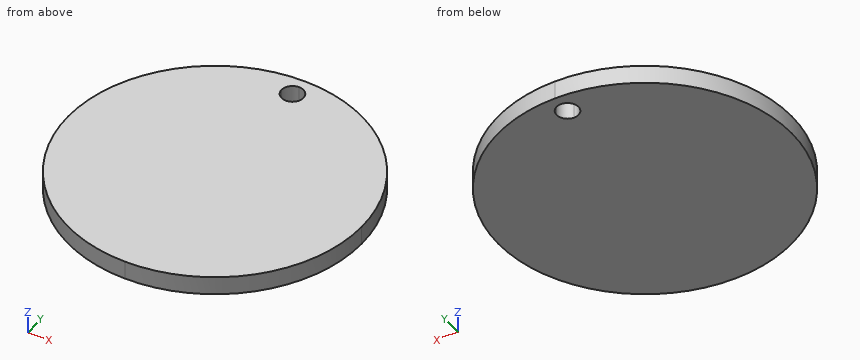
```python
from build123d import *

# Parameters (mm, degrees)
F1_DEPTH = 6.35


with BuildPart() as f1:
    # F0 (on Top) → F1 (new body)
    with BuildSketch(Plane.XY):
        with BuildLine():
            Line((0, 47.5154318641), (0, 50.8))
            ThreePointArc((0, 50.8), (-50.8, 0), (0, -50.8))
            Line((0, -50.8), (0, 39.9495042134))
            ThreePointArc((0, 39.9495042134), (-2.6749593739, 41.0575086649), (-3.7829638253, 43.7324680388))
            ThreePointArc((-3.7829638253, 43.7324680388), (-2.6749593739, 46.4074274127), (0, 47.5154318641))
        make_face()
        with BuildLine():
            ThreePointArc((0, -50.8), (35.9210244843, -35.9210244843), (50.8, 0))
            ThreePointArc((50.8, 0), (35.9210244843, 35.9210244843), (0, 50.8))
            Line((0, 50.8), (0, 47.5154318641))
            ThreePointArc((0, 47.5154318641), (2.6749593739, 46.4074274127), (3.7829638253, 43.7324680388))
            ThreePointArc((3.7829638253, 43.7324680388), (2.6749593739, 41.0575086649), (0, 39.9495042134))
            Line((0, 39.9495042134), (0, -50.8))
        make_face()
    extrude(amount=F1_DEPTH)


solid = f1.part
```
For this review, take the finished solid that the model builds, in its own axes (mm). Give positions to 0.01 mm unless a question says otherwise; leave off trailing zeros. Write each loop counter-clockwise with the first axis right and the second up, starting at its lowest first coordinate (ties: lowest second). Pieces come first, ordered by that corner, then holes. Notation, with made-up numbers: M -27.75,50.5 L -20.75,50.5 A24 cw -20.75,76.5 Z; hole C -3,9.5 d10. An arc over 180 degrees is marked long. One line per item, written item: value.
1) Take a section at C-C, the plane x = 37.5. Write out the cut boundary in (y, z), then the cut area to 3 significant figures.
Results are:
outline: M -34.27,0 L 34.27,0 L 34.27,6.35 L -34.27,6.35 Z
area: 435 mm²
2) Take a section at B-B, the plane y = 41.5. Write out the cut boundary in (x, z), then the cut area to 3 significant figures.
Results are:
outline: M -29.3,0 L -3.05,0 L -3.05,6.35 L -29.3,6.35 Z; M 3.05,0 L 29.3,0 L 29.3,6.35 L 3.05,6.35 Z
area: 333 mm²
3) Take a section at A-A, the plane z = 2.5. Write out the cut boundary in (x, y), then the cut area to 3 significant figures.
Results are:
outline: C 0,0 d101.6; hole C 0,43.73 d7.57
area: 8,060 mm²
4) Take a section at D-D, the plane y = 17.5. Write out the cut boundary in (x, z).
Results are:
outline: M -47.69,0 L 47.69,0 L 47.69,6.35 L -47.69,6.35 Z
5) For line 1 (X direction, y = -1, z = 2.25); line 2 (Y direction, x = -1.5, z = 4.5); line 3 (Y direction, x = -2, z = 4), list the stretches that pass through material, from the lowest coordinate up. Write a range as from..to.
Results are:
line 1: x = -50.79..50.79
line 2: y = -50.78..40.26, 47.21..50.78
line 3: y = -50.76..40.52, 46.94..50.76
6) For P1, Ø1, axis at x = -14.5, y = -34.5, coming from the -Z side; P2, Ø1.5, axis at x = 38, z = 1, coming from the -Y side, all flat-tipped, find the tip position at first contact; note any pin that passes through.
Results are:
P1: stops at z = 0
P2: stops at y = -34.54
